Here's how the part is built. I have some questions about the finished solid (model axes, mm). Face numbers are marked on the shaded views. A direction names the side the tool comes from. Round coordinates to 2 decimals unless told otherwise and drop trailing zeros. Write each loop counter-clockwise with the first axis right and the second up, starting at its lowest first coordinate (ties: lowest second). Pieces come first, ordered by that corner, then holes. Notation, with made-up numbers: (76, 55.5) - (127, 55.5) arc R12 ccw to (127, 74.5) - close; hole circle Ø7 at (-11.75, 75.25). An arc over 180 degrees is marked (long way). One line per item, written item: value. Start each with the question number.
Item 1: For P1, Ø5, axis at y = -90, z = 8, coming from the +X side; P2, Ø1.5, axis at x = 13, y = -21.5, coming from the +Z side; P3, Ø1.5, axis at y = -15, z = 11, coming from the -X side, each with a flat end and sliding along its axis, tell me the tip position at first contact or that it passes through.
Item 2: If I drill on line 1 (Z direction, x = -0.5, y = -72.5); line 2 (Z direction, x = 9, y = -93); line 3 (Y direction, x = -10, z = -11), over which ranges is the centre line in solid material (lowest first)?
Item 3: Imagine slicing it at C-C, the plane y = -106.5. Please give me the cut outline in (x, z), then the cut area to 3 significant figures.
Item 4: For the marked faces 1 and 2, which set-ups out of +Z, -Z, +X, -X, +Y, -Y let a thin tool reach every point of the face, with its end or its side?
Item 5: Imagine slicing it at A-A, the plane x = 0. Please give me the cut outline in (y, z).
Item 6: Imagine slicing it at B-B, the plane y = -2. Please give me the cut outline in (x, z).
```python
from build123d import *

# Parameters (mm, degrees)
SKETCH2_W          = 5
SKETCH2_H          = 120
CUT_EXTRUDE1_START = -25
CUT_EXTRUDE1_DEPTH = 25
FILLET1_R          = 3


with BuildPart() as part:
    # Sketch1 → Revolve1 (revolve)
    with BuildSketch(Plane.XY, mode=Mode.PRIVATE) as revolve1_sk:
        with BuildLine():
            Line((0, -150), (15, -150))
            Line((15, -150), (15, 0))
            Line((15, 0), (21, 0))
            Line((21, 0), (9.396926208, 31.87918324))
            ThreePointArc((9.396926208, 31.87918324), (5.735764364, 36.65050225), (0, 38.458981807))
            Line((0, 38.458981807), (0, -150))
        make_face()
    revolve(revolve1_sk.sketch.rotate(Axis((0, -160.189242242, 0), (0, 1, 0)), 90), axis=Axis((0, -160.189242242, 0), (0, 1, 0)))

    # Sketch2 → Cut-Revolve1 (revolve, cut)
    with BuildSketch(Plane.XY):
        with Locations((12.5, -90)):
            Rectangle(SKETCH2_W, SKETCH2_H)
    revolve(axis=Axis((0, 9.42117093, 0), (0, -1, 0)), mode=Mode.SUBTRACT)

    # Sketch3 → Cut-Extrude1 (cut)
    with BuildSketch(Plane.XZ.offset(30).offset(CUT_EXTRUDE1_START)):
        with BuildLine():
            Line((14.696938457, 3), (11.696938457, 3))
            Line((11.696938457, 3), (11.696938457, -3))
            Line((11.696938457, -3), (14.696938457, -3))
            ThreePointArc((14.696938457, -3), (15, 0), (14.696938457, 3))
        make_face()
    extrude(amount=CUT_EXTRUDE1_DEPTH, mode=Mode.SUBTRACT)

    # Fillet1
    fillet1_edges = [part.edges().sort_by_distance(p)[0] for p in [
        (13.196938457, -5, 3),
        (13.196938457, -5, -3),
    ]]
    fillet(fillet1_edges, radius=FILLET1_R - 0.0001)  # a hair under: the kernel refuses the full size


solid = part.part
```
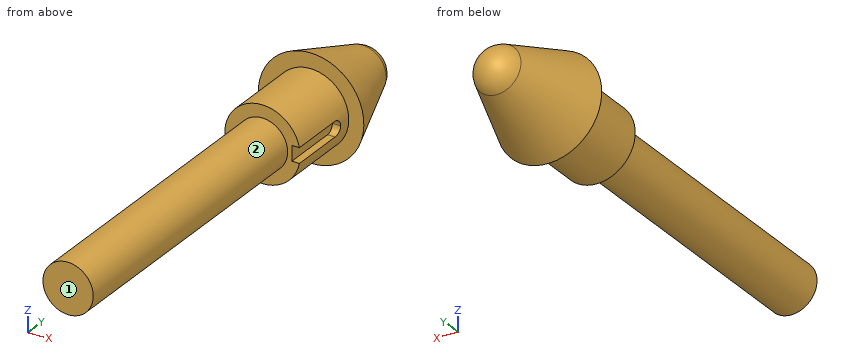
Values follow:
1. P1: stops at x = 8.35
1. P2: stops at z = 8.66
1. P3: stops at x = -10.95
2. line 1: z = -9.99 to 9.99
2. line 2: z = -4.36 to 4.36
2. line 3: y = -30 to 16.85
3. outline: circle Ø20 at (0, 0)
3. area: 314 mm^2
4. face 1: +Z, -Z, +X, -X, -Y
4. face 2: -Y
5. outline: (-150, -10) - (-30, -10) - (-30, -15) - (0, -15) - (0, -21) - (31.88, -9.4) arc R10 ccw to (31.88, 9.4) - (0, 21) - (0, 15) - (-30, 15) - (-30, 10) - (-150, 10) - close
6. outline: circle Ø30 at (0, 0)
